```python
from build123d import *

# Parameters (mm, degrees)
EXTRUDE_1_DEPTH     = 80
SKETCH_2_W          = 15
SKETCH_2_H          = 15
CUT_EXTRUDE_1_DEPTH = 35
SKETCH_3_R          = 4
CUT_EXTRUDE_2_DEPTH = 93.870878105
CUT_EXTRUDE_START   = -35
CUT_EXTRUDE_4_DEPTH = 35
FILLET_1_R          = 1
EXTRUDE_START       = -5
EXTRUDE_2_DEPTH     = 5


with BuildPart() as part:
    # 草图1 → 凸台-拉伸1 (new body)
    with BuildSketch(Plane.XY):
        with BuildLine():
            Line((-20, 15), (-20, -15))
            ThreePointArc((-20, -15), (0, -25), (20, -15))
            Line((20, -15), (20, 15))
            ThreePointArc((20, 15), (0, 25), (-20, 15))
        make_face()
    extrude(amount=EXTRUDE_1_DEPTH)

    # 草图2 → 切除-拉伸1 (cut)
    with BuildSketch(Plane(origin=(0, 0, 0), x_dir=(-1, 0, 0), z_dir=(0, 0, -1))):
        Rectangle(SKETCH_2_W, SKETCH_2_H)
    extrude(amount=-CUT_EXTRUDE_1_DEPTH, mode=Mode.SUBTRACT)

    # 草图3 → 切除-拉伸2 (cut, through all)
    with BuildSketch(Plane.ZY.offset(20)):
        with Locations((8, 0)):
            Circle(SKETCH_3_R)
        with Locations((27, 0)):
            Circle(SKETCH_3_R)
        with Locations((60, 9.5)):
            Circle(SKETCH_3_R)
        with Locations((60, -9.5)):
            Circle(SKETCH_3_R)
    extrude(amount=-CUT_EXTRUDE_2_DEPTH, mode=Mode.SUBTRACT)

    # 草图6 → 切除-拉伸4 (cut)
    with BuildSketch(Plane.XY.offset(80).offset(CUT_EXTRUDE_START)):
        with BuildLine():
            Line((-20, 15), (20, 15))
            ThreePointArc((20, 15), (0, 25), (-20, 15))
        make_face()
    extrude(amount=CUT_EXTRUDE_4_DEPTH, mode=Mode.SUBTRACT)

    # 圆角1
    fillet_1_edges = [part.edges().sort_by_distance(p)[0] for p in [
        (7.5, -7.5, 17.5),
        (7.5, 7.5, 17.5),
        (-7.5, 7.5, 17.5),
        (-7.5, -7.5, 17.5),
    ]]
    fillet(fillet_1_edges, radius=FILLET_1_R)

    # 草图6<2> → 凸台-拉伸2 (add)
    with BuildSketch(Plane.XY.offset(80).offset(EXTRUDE_START)):
        with BuildLine():
            Line((-20, 15), (20, 15))
            ThreePointArc((20, 15), (0, 25), (-20, 15))
        make_face()
    extrude(amount=EXTRUDE_2_DEPTH)


solid = part.part
```
The model under review builds one solid part; all positions refer to its coordinate system, in mm. A direction names the side the tool comes from. Round coordinates to 2 decimals unless told otherwise and drop trailing zeros. Loops run counter-clockwise (first coordinate to the right, second up) from the corner with the lowest first, then second, coordinate; pieces in that order, holes last.
1) Consider section D-D on z = 60. State the section outline as (x, y) points.
Values follow:
outline: (-20, -15) arc R25 ccw to (20, -15) - (20, -13.5) - (-20, -13.5) - close; (-20, -5.5) - (20, -5.5) - (20, 5.5) - (-20, 5.5) - close; (-20, 13.5) - (20, 13.5) - (20, 15) - (-20, 15) - close
2) Consider section B-B on y = -9.5. State the section outline as (x, z) points, then the cut area to 3 significant figures.
Values follow:
outline: (-20, 0) - (20, 0) - (20, 56) - (-20, 56) - close; (-20, 64) - (20, 64) - (20, 80) - (-20, 80) - close
area: 2,880 mm2
3) Tool access review of faces 1 (the face through (0, 19, 45)), 2 (the face through (7.5, 0, 17)), 3 (the face through (-20, 0, 39)): name each direction out of +Z, -Z, +X, -X, +Y, -Y from which nothing blocks a thin tool from reaching the whole face with its end or side.
Values follow:
face 1: +X, -X, +Y
face 2: -Z
face 3: +Z, -Z, -X, +Y, -Y
4) Wall thickness on line 1 along X through (y, z) = (3.5, 20); line 2 along Y through (x, z) = (15, 8); line 3 along Z through (x, y) = (-9.5, 1): over which ranges is each line inside the solid? List them lowest first.
Values follow:
line 1: x = -20 to -7.5, 7.5 to 20
line 2: y = -20 to -4, 4 to 20
line 3: z = 0 to 4.13, 11.87 to 23.13, 30.87 to 80
5) Consider section A-A on y = 0. State the section outline as (x, z) points.
Values follow:
outline: (-20, 0) - (-7.5, 0) - (-7.5, 4) - (-20, 4) - close; (-20, 12) - (-7.5, 12) - (-7.5, 23) - (-20, 23) - close; (-20, 31) - (-7.5, 31) - (-7.5, 35) - (7.5, 35) - (7.5, 31) - (20, 31) - (20, 80) - (-20, 80) - close; (7.5, 0) - (20, 0) - (20, 4) - (7.5, 4) - close; (7.5, 12) - (20, 12) - (20, 23) - (7.5, 23) - close
6) Consider section C-C on z = 27. State the section outline as (x, y) points.
Values follow:
outline: (-20, -15) arc R25 ccw to (20, -15) - (20, -4) - (7.5, -4) - (7.5, -6.5) arc R1 cw to (6.5, -7.5) - (-6.5, -7.5) arc R1 cw to (-7.5, -6.5) - (-7.5, -4) - (-20, -4) - close; (-20, 4) - (-7.5, 4) - (-7.5, 6.5) arc R1 cw to (-6.5, 7.5) - (6.5, 7.5) arc R1 cw to (7.5, 6.5) - (7.5, 4) - (20, 4) - (20, 15) arc R25 ccw to (-20, 15) - close
7) The part is to be moulded in two halves that separate along X. For faces 4 (the face through (-7.5, 0, 17)), 5 (the face through (0, -25, 39)), 6 (the face through (0, 19, 75)), say which applies: pulls with the +X half, pulls with the -X half, needs draft (parallel to the pull), parting line crosses it, or undercut.
Values follow:
face 4: undercut
face 5: parting line crosses it
face 6: needs draft
8) Clearance check with flat-ended pins moving along their axes: P1, Ø4, axis at y = -0.5, z = 28, coming from the +X side; P2, Ø1.5, axis at x = -16, z = 18.5, coming from the -Y side; P3, Ø12, axis at x = 12.5, z = 67, coming from the +Y side; P4, Ø5, axis at x = 5.5, z = 32, coming from the -Y side. State where each tip first meets the part, or that it passes through.
Values follow:
P1: passes through
P2: stops at y = -19.81
P3: stops at y = 15
P4: stops at y = -24.82
